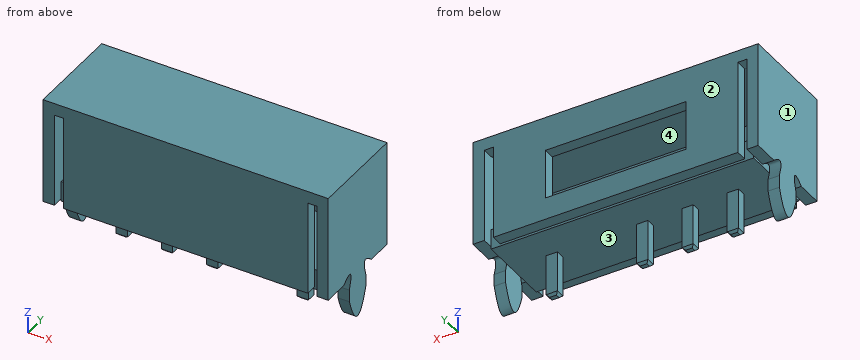
```python
from build123d import *

# Parameters (mm, degrees)
SKETCH_1_W           = 12.6
SKETCH_1_H           = 4.3
SKETCH_1_W_2         = 11.6
SKETCH_1_H_2         = 3.3
EXTRUDE_1_DEPTH      = 4.7
SKETCH_4_W           = 11.6
SKETCH_4_H           = 3.3
EXTRUDE_3_DEPTH      = 0.5
SKETCH_6_W           = 0.4
SKETCH_6_H           = 4.166312425
CUT_EXTRUDE_2_DEPTH  = 9.959352655
EXTRUDE_4_DEPTH      = 0.8
EXTRUDE_4_DEPTH_BACK = 0.1
SKETCH_7_W           = 11.6
SKETCH_7_H           = 3.3
EXTRUDE_START        = -0.1
SKETCH_8_W           = 0.5
SKETCH_8_H           = 0.4
EXTRUDE_5_DEPTH      = 2
SKETCH_9_W           = 6.2
SKETCH_9_H           = 2.2
CUT_EXTRUDE_3_DEPTH  = 0.5
CUT_EXTRUDE_4_DEPTH  = 0.5
CUT_EXTRUDE_START    = -12.6
CUT_EXTRUDE_5_DEPTH  = 0.5
CHAMFER_1_SIZE       = 0.1


with BuildPart() as part:
    # Sketch 1 → Extrude 1 (new body)
    with BuildSketch(Plane.XY):
        Rectangle(SKETCH_1_W, SKETCH_1_H)
        Rectangle(SKETCH_1_W_2, SKETCH_1_H_2, mode=Mode.SUBTRACT)
    extrude(amount=EXTRUDE_1_DEPTH)

    # Sketch 4 → Extrude 3 (add)
    with BuildSketch(Plane.XY.offset(4.7)):
        Rectangle(SKETCH_4_W, SKETCH_4_H)
    extrude(amount=-EXTRUDE_3_DEPTH)

    # Sketch 6 → Cut-Extrude 2 (cut, through all)
    with BuildSketch(Plane.XZ.offset(2.15)):
        with Locations((-5.6, 2.083156213)):
            Rectangle(SKETCH_6_W, SKETCH_6_H)
        with Locations((5.6, 2.083156213)):
            Rectangle(SKETCH_6_W, SKETCH_6_H)
    extrude(amount=-CUT_EXTRUDE_2_DEPTH, mode=Mode.SUBTRACT)



with BuildPart() as body_2:
    # Sketch 7 → Extrude 4 (new, two sides: drawn at the far end of the back side and taken through both)
    with BuildSketch(Plane.XY.offset(-EXTRUDE_4_DEPTH_BACK)):
        Rectangle(SKETCH_7_W, SKETCH_7_H)
    extrude(amount=EXTRUDE_4_DEPTH + EXTRUDE_4_DEPTH_BACK)


with BuildPart() as part_1:
    add(part.part)

    add(body_2.part)  # Extrude 5 merges body 2
    # Sketch 8 → Extrude 5 (add)
    with BuildSketch(Plane(origin=(0, 0, -0.1), x_dir=(-1, 0, 0), z_dir=(0, 0, -1)).offset(EXTRUDE_START)):
        with Locations((4, 0)):
            Rectangle(SKETCH_8_W, SKETCH_8_H)
        with Locations((2, 0)):
            Rectangle(SKETCH_8_W, SKETCH_8_H)
        Rectangle(SKETCH_8_W, SKETCH_8_H)
        with Locations((-4, 0)):
            Rectangle(SKETCH_8_W, SKETCH_8_H)
        Polygon((-5.8, 0), (-5.8, 0.6), (-6.3, 0.6), (-6.3, -0.6), (-5.8, -0.6), align=None)
        Polygon((5.8, -0.6), (5.8, 0), (5.8, 0.6), (6.3, 0.6), (6.3, -0.6), align=None)
    extrude(amount=EXTRUDE_5_DEPTH)

    # Sketch 9 → Cut-Extrude 3 (cut)
    with BuildSketch(Plane(origin=(0, 2.15, 0), x_dir=(1, 0, 0), z_dir=(0, 1, 0))):
        with Locations((0, -2.083156212)):
            Rectangle(SKETCH_9_W, SKETCH_9_H)
    extrude(amount=-CUT_EXTRUDE_3_DEPTH, mode=Mode.SUBTRACT)

    # Sketch 10 → Cut-Extrude 4 (cut)
    with BuildSketch(Plane(origin=(6.3, 0, 0), x_dir=(0, 0, -1), z_dir=(1, 0, 0))):
        with BuildLine():
            Line((0, 1.000258095), (0.460284105, 0.6))
            add(Edge.make_bspline(
                [(0.460284105, 0.6), (-0.677187697, 0.248999902), (0, 1.000258095)],
                knots=[0, 0, 0, 1, 1, 1], degree=2))
        make_face()
        with BuildLine():
            Line((0.460284105, -0.6), (0, -1.000258095))
            add(Edge.make_bspline(
                [(0.460284105, -0.6), (-0.677187697, -0.248999902), (0, -1.000258095)],
                knots=[0, 0, 0, 1, 1, 1], degree=2))
        make_face()
        with BuildLine():
            Line((1, 0.6), (4, 0.6))
            Line((4, 0.6), (4.247891551, 0.6))
            Line((4.247891551, 0.6), (4.247891551, -0.6))
            Line((4.247891551, -0.6), (1, -0.6))
            add(Edge.make_bspline(
                [(1, 0.6), (3, 0), (1, -0.6)],
                knots=[0, 0, 0, 1, 1, 1], degree=2))
        make_face()
    extrude(amount=-CUT_EXTRUDE_4_DEPTH, mode=Mode.SUBTRACT)

    # Sketch 10_2 → Cut-Extrude 5 (cut)
    with BuildSketch(Plane(origin=(6.3, 0, 0), x_dir=(0, 0, -1), z_dir=(1, 0, 0)).offset(CUT_EXTRUDE_START)):
        with BuildLine():
            Line((0, 1.000258095), (0.460284105, 0.6))
            add(Edge.make_bspline(
                [(0.460284105, 0.6), (-0.677187697, 0.248999902), (0, 1.000258095)],
                knots=[0, 0, 0, 1, 1, 1], degree=2))
        make_face()
        with BuildLine():
            Line((0.460284105, -0.6), (0, -1.000258095))
            add(Edge.make_bspline(
                [(0.460284105, -0.6), (-0.677187697, -0.248999902), (0, -1.000258095)],
                knots=[0, 0, 0, 1, 1, 1], degree=2))
        make_face()
        with BuildLine():
            Line((1, 0.6), (4, 0.6))
            Line((4, 0.6), (4.247891551, 0.6))
            Line((4.247891551, 0.6), (4.247891551, -0.6))
            Line((4.247891551, -0.6), (1, -0.6))
            add(Edge.make_bspline(
                [(1, 0.6), (3, 0), (1, -0.6)],
                knots=[0, 0, 0, 1, 1, 1], degree=2))
        make_face()
    extrude(amount=CUT_EXTRUDE_5_DEPTH, mode=Mode.SUBTRACT)

    # Chamfer 1
    chamfer_1_edges = [part_1.edges().sort_by_distance(p)[0] for p in [
        (-4, 0.2, -2),
        (-3.75, 0, -2),
        (-4, -0.2, -2),
        (-4.25, 0, -2),
        (-2, 0.2, -2),
        (-1.75, 0, -2),
        (-2, -0.2, -2),
        (-2.25, 0, -2),
        (4, 0.2, -2),
        (4.25, 0, -2),
        (4, -0.2, -2),
        (3.75, 0, -2),
        (0, 0.2, -2),
        (0.25, 0, -2),
        (0, -0.2, -2),
        (-0.25, 0, -2),
    ]]
    chamfer(chamfer_1_edges, length=CHAMFER_1_SIZE)


solid = part_1.part
```
Geometry: final body of the model. Coordinates: model frame, mm. Face numbers are marked on the shaded views. Round coordinates to 2 decimals unless told otherwise and drop trailing zeros. Order: outer loops, then holes, each group sorted by start corner. A loop starts at its lowest first (then second) coordinate and runs counter-clockwise, first axis right, second up. Notation, with made-up numbers: M 9.5,-7.75 L 43.5,-7.75 A11 ccw 43.5,0.25 Z; hole C 27,72.5 d6. An arc over 180 degrees is marked long. One line per item, written item: value.
(1) Cut plane C-C (y = -1.9). Return the cut outline in (x, z).
Result sheet:
outline: M -6.3,0 L -5.8,0 L -5.8,4.17 L -5.4,4.17 L -5.4,0 L 5.4,0 L 5.4,4.17 L 5.8,4.17 L 5.8,0 L 6.3,0 L 6.3,4.7 L -6.3,4.7 Z
(2) Cut plane D-D (y = 1.4). Return the cut outline in (x, z).
Result sheet:
outline: M -6.3,0 L -5.8,0 L -5.8,-0.1 L 5.8,-0.1 L 5.8,0 L 6.3,0 L 6.3,4.7 L -6.3,4.7 Z; hole M -5.8,0.8 L 5.8,0.8 L 5.8,4.2 L -5.8,4.2 Z
(3) Pin query (flat end, axial travel): P1, Ø1.7, axis at x = 2, z = 2, coming from the +Y side; P2, Ø0.6, axis at x = -6, z = -0.5, coming from the -Y side; P3, Ø2, axis at x = 2.5, y = -1, coming from the -Z side. Return the tip coordinate at first contact, or that it passes through.
Result sheet:
P1: y = -1.65
P2: y = -0.6
P3: z = -0.1
(4) Line query: probe 1 along X at (y, z) = (-0.05, -0.75); probe 2 along X at (y, z) = (-1.75, 1.25); probe 3 along Z at (x, y) = (1.5, 1). Output: solid intervals per line, ascending. Write a range as [from, to].
Result sheet:
probe 1: [-6.3, -5.8], [-4.25, -3.75], [-2.25, -1.75], [-0.25, 0.25], [3.75, 4.25], [5.8, 6.3]
probe 2: [-6.3, -5.8], [-5.4, 5.4], [5.8, 6.3]
probe 3: [-0.1, 0.8], [4.2, 4.7]
(5) Cut plane B-B (x = 5.25). Return the cut outline in (y, z), and give its area (3 significant figures).
Result sheet:
outline: M -2.15,0 L -1.65,0 L -1.65,-0.1 L 1.65,-0.1 L 1.65,0 L 2.15,0 L 2.15,4.7 L -2.15,4.7 Z; hole M -1.65,0.8 L 1.65,0.8 L 1.65,4.2 L -1.65,4.2 Z
area: 9.32 mm2
(6) Pull-direction query (X, two-part tool) for the marked faces 1, 2, 3 and 4; classes: pulls with the +X half, pulls with the -X half, needs draft (parallel to the pull), parting line crosses it, or undercut.
Result sheet:
face 1: pulls with the -X half
face 2: needs draft
face 3: undercut
face 4: undercut
(7) Cut plane A-A (z = 2.5). Return the cut outline in (x, y).
Result sheet:
outline: M -6.3,-2.15 L -5.8,-2.15 L -5.8,2.15 L -6.3,2.15 Z; M -5.4,-2.15 L 5.4,-2.15 L 5.4,-1.65 L -5.4,-1.65 Z; M -5.4,1.65 L -3.1,1.65 L -3.1,2.15 L -5.4,2.15 Z; M 3.1,1.65 L 5.4,1.65 L 5.4,2.15 L 3.1,2.15 Z; M 5.8,-2.15 L 6.3,-2.15 L 6.3,2.15 L 5.8,2.15 Z
